```python
from build123d import *

# Parameters (mm, degrees)
SKETCH1_R           = 15
SKETCH1_R_2         = 0.75
BOSS_EXTRUDE1_DEPTH = 3
FILLET1_R           = 2


with BuildPart() as part:
    # Sketch1 → Boss-Extrude1 (new body)
    with BuildSketch(Plane(origin=(0, 0, 0), x_dir=(1, 0, 0), z_dir=(0, 1, 0))):
        Circle(SKETCH1_R)
        with Locations((0, 10.5)):
            Circle(SKETCH1_R_2, mode=Mode.SUBTRACT)
        with Locations((0, 7)):
            Circle(SKETCH1_R_2, mode=Mode.SUBTRACT)
        with Locations((0, 3.5)):
            Circle(SKETCH1_R_2, mode=Mode.SUBTRACT)
        with Locations((3.031088913, 1.75)):
            Circle(SKETCH1_R_2, mode=Mode.SUBTRACT)
        with Locations((6.062177826, 3.5)):
            Circle(SKETCH1_R_2, mode=Mode.SUBTRACT)
        with Locations((9.09326674, 5.25)):
            Circle(SKETCH1_R_2, mode=Mode.SUBTRACT)
        with Locations((3.031088913, -1.75)):
            Circle(SKETCH1_R_2, mode=Mode.SUBTRACT)
        with Locations((6.062177826, -3.5)):
            Circle(SKETCH1_R_2, mode=Mode.SUBTRACT)
        with Locations((9.09326674, -5.25)):
            Circle(SKETCH1_R_2, mode=Mode.SUBTRACT)
        with Locations((0, -3.5)):
            Circle(SKETCH1_R_2, mode=Mode.SUBTRACT)
        with Locations((0, -7)):
            Circle(SKETCH1_R_2, mode=Mode.SUBTRACT)
        with Locations((0, -10.5)):
            Circle(SKETCH1_R_2, mode=Mode.SUBTRACT)
        with Locations((-3.031088913, -1.75)):
            Circle(SKETCH1_R_2, mode=Mode.SUBTRACT)
        with Locations((-6.062177826, -3.5)):
            Circle(SKETCH1_R_2, mode=Mode.SUBTRACT)
        with Locations((-9.09326674, -5.25)):
            Circle(SKETCH1_R_2, mode=Mode.SUBTRACT)
        with Locations((-3.031088913, 1.75)):
            Circle(SKETCH1_R_2, mode=Mode.SUBTRACT)
        with Locations((-6.062177826, 3.5)):
            Circle(SKETCH1_R_2, mode=Mode.SUBTRACT)
        with Locations((-9.09326674, 5.25)):
            Circle(SKETCH1_R_2, mode=Mode.SUBTRACT)
    extrude(amount=BOSS_EXTRUDE1_DEPTH)

    # Fillet1
    fillet1_edges = [part.edges().sort_by_distance(p)[0] for p in [
        (-15, 3, 0),
    ]]
    fillet(fillet1_edges, radius=FILLET1_R)


solid = part.part
```
Part model, mm, in its own coordinate system. Round coordinates to 2 decimals unless told otherwise and drop trailing zeros.
1. Two-plate mould, pull along Z, no slides. Class faces 1 (the face through (0, 0, 0)), 2 (the face through (5.9, 1.479, 4.232)): pulls with the +Z half, pulls with the -Z half, needs draft (parallel to the pull), parting line crosses it, or undercut.
Solutions:
face 1: needs draft
face 2: undercut
2. Slice it at A-A (y = 1.55). Count the separate pieces of the cut face and the enclosed holes in it, and give its area (3 significant figures).
Solutions:
separate pieces: 1
enclosed holes: 18
area: 668 mm2
3. Flat gauge pin, fed straight in: pin 1 (2.5 mm diameter, centred on x = -3.03, z = -1.75, fed in from +Y). Where does the tip first touch, or does it go through?
Solutions:
pin 1: stops at y = 3
4. Drill centre lines: line 1 along X through (y, z) = (2.1, -1.75); line 2 along X through (y, z) = (1.3, -5.25); line 3 along Z through (x, y) = (3.5, 1.6). Where is each one in solid material? Low to high.
Solutions:
line 1: x = -14.57 to -3.78, -2.28 to 2.28, 3.78 to 14.57
line 2: x = -14.03 to -9.84, -8.34 to 8.34, 9.84 to 14.03
line 3: z = -14.49 to -2.34, -1.16 to 1.16, 2.34 to 14.49
